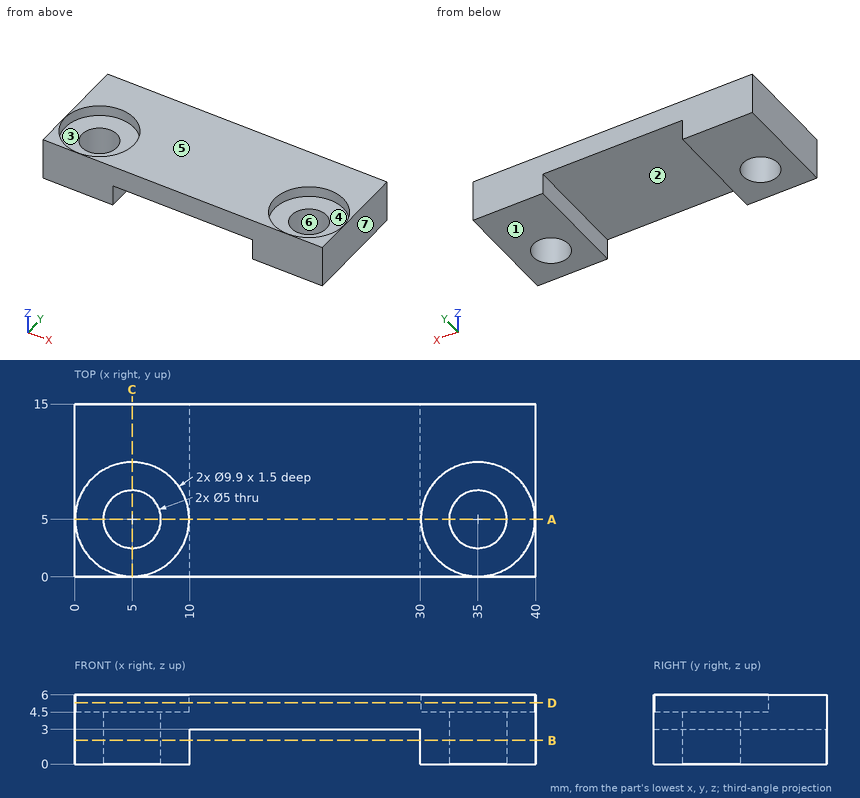
Print and shaded views of the part. All mm, measured from the part's lowest x, y and z. A direction names the side the tool comes from. Give positions to 0.01 mm unless a question says otherwise; leave off trailing zeros. Loops run counter-clockwise (first coordinate to the right, second up) from the corner with the lowest first, then second, coordinate; pieces in that order, holes last. Notation, with made-up numbers: (-6, 53) - (36, 53) arc R9 ccw to (36, 61) - close; hole circle Ø4 at (53.5, 38.25). An arc over 180 degrees is marked (long way). Use a Markdown table: item, result.
(1) Band-saw the part on A-A (y = 5). Give the cut face in (x, z), and give its area (3 significant figures).
Taken from the geometry:
| item | result |
|---|---|
| outline | (0, 0) - (2.5, 0) - (2.5, 4.5) - (0.05, 4.5) - (0.05, 6) - (0, 6) - close; (7.5, 0) - (10, 0) - (10, 3) - (30, 3) - (30, 0) - (32.5, 0) - (32.5, 4.5) - (30.05, 4.5) - (30.05, 6) - (9.95, 6) - (9.95, 4.5) - (7.5, 4.5) - close; (37.5, 0) - (40, 0) - (40, 6) - (39.95, 6) - (39.95, 4.5) - (37.5, 4.5) - close |
| area | 105 mm2 |
(2) Band-saw the part on B-B (z = 2.05). Give the cut face in (x, y).
Taken from the geometry:
| item | result |
|---|---|
| outline | (0, 0) - (10, 0) - (10, 15) - (0, 15) - close; (30, 0) - (40, 0) - (40, 15) - (30, 15) - close; hole circle Ø5 at (5, 5); hole circle Ø5 at (35, 5) |
(3) Pull direction X, two halves, no side cores. Call the marked faces 4, 5, 6 and 7: +X half, -X half, draft (parallel to the pull), parting line (faces both ways), or undercut.
Taken from the geometry:
| item | result |
|---|---|
| face 4 | undercut |
| face 5 | draft |
| face 6 | undercut |
| face 7 | +X half |
(4) Band-saw the part on D-D (z = 5.3). Give the cut face in (x, y).
Taken from the geometry:
| item | result |
|---|---|
| outline | (0, 0) - (40, 0) - (40, 15) - (0, 15) - close; hole circle Ø9.9 at (5, 5); hole circle Ø9.9 at (35, 5) |
(5) Drop a flat-ended pin along its axis: pin 1 Ø6 at (x, y) = (35, 5) entering from +Z. Give the stop position or say it passes through.
Taken from the geometry:
| item | result |
|---|---|
| pin 1 | z = 4.5 |
(6) Band-saw the part on C-C (x = 5). Give the cut face in (y, z), and give its area (4 significant figures).
Taken from the geometry:
| item | result |
|---|---|
| outline | (0, 0) - (2.5, 0) - (2.5, 4.5) - (0.05, 4.5) - (0.05, 6) - (0, 6) - close; (7.5, 0) - (15, 0) - (15, 6) - (9.95, 6) - (9.95, 4.5) - (7.5, 4.5) - close |
| area | 52.65 mm2 |
(7) Wall check: line 1 along X through (y, z) = (6.75, 2.1); line 2 along X through (y, z) = (13, 2.85); line 3 along X through (y, z) = (1.75, 4.95). Give the ranges that are in metal, low to high.
Taken from the geometry:
| item | result |
|---|---|
| line 1 | 0 to 3.21, 6.79 to 10, 30 to 33.21, 36.79 to 40 |
| line 2 | 0 to 10, 30 to 40 |
| line 3 | 0 to 1.27, 8.73 to 31.27, 38.73 to 40 |
(8) Which spindle directions (+Z, -Z, +X, -X, +Y, -Y) get a long thin tool onto all of the face, cutting with end or side? Do the marked faces 1, 2 and 3. Say none if no direction does.
Taken from the geometry:
| item | result |
|---|---|
| face 1 | -Z, +X, -X, +Y, -Y |
| face 2 | -Z, +Y, -Y |
| face 3 | +Z |
